Autodesk Inventor part; units mm, degrees
ref_plane "YZ Plane" through (0, 0, 0) normal (1, 0, 0) x (0, 1, 0)
ref_plane "XZ Plane" through (0, 0, 0) normal (0, 1, 0) x (-1, 0, 0)
ref_plane "XY Plane" through (0, 0, 0) normal (0, 0, 1) x (1, 0, 0)
sketch "Sketch1" plane through (0, 0, 0) normal (0, 1, 0) x (-1, 0, 0)
  circle A0 centre (0, 0) radius 7.5
  circle A1 centre (0, -10.775) radius 1.725
  circle A2 centre (0, 10.775) radius 1.725
  line L0 (8.1017, 5.1965) -> (3.205, 12.8307)
  line L1 (-3.205, 12.8307) -> (-8.1017, 5.1965)
  line L2 (-8.1017, -5.1965) -> (-3.205, -12.8307)
  line L3 (3.205, -12.8307) -> (8.1017, -5.1965)
  line L4 (0, -20) -> (0, 18) construction
  arc A3 (-3.205, -12.8307) -> (3.205, -12.8307) centre (0, -10.775) ccw
  arc A4 (8.1017, -5.1965) -> (8.1017, 5.1965) centre (0, 0) ccw
  arc A5 (-8.1017, 5.1965) -> (-8.1017, -5.1965) centre (0, 0) ccw
  arc A6 (3.205, 12.8307) -> (-3.205, 12.8307) centre (0, 10.775) ccw
  dimension "d0" = 15
  dimension "d2" = 3.45
  dimension "d4" = 10.775
  dimension "d8" = 3.45
  dimension "d9" = 10.775
  dimension "d34" = 9.625
  dimension "d35" = 9.625
extrude "Extrusion1" add sketch "Sketch1" along normal blind 1.25 contours A0 | A4 L3 A3 L2 A5 L1 A6 L0
fillet "Fillet1" radius 1.25 8 edges at (5.6534, 1.25, 9.0136) (9.625, 1.25, 0) (5.6534, 1.25, -9.0136) (0, 1.25, -14.5826) (-5.6534, 1.25, -9.0136) (-9.625, 1.25, 0) (-5.6534, 1.25, 9.0136) (0, 1.25, 14.5826)
extrude "Extrusion2" add sketch "Sketch1" against normal blind 11.3 contours A0
fillet "Fillet2" radius 1.25 1 edges at (7.5, -11.3, 0)
sketch "Sketch2" plane through (0, -11.3, 0) normal (0, -1, 0) x (1, 0, 0)
  circle A0 centre (0, 0) radius 3.26 construction
  line L0 (-0.25, -2.26) -> (0.25, -2.26)
  line L1 (0.25, -2.26) -> (0.25, -4.26)
  line L2 (0.25, -4.26) -> (-0.25, -4.26)
  line L3 (-0.25, -4.26) -> (-0.25, -2.26)
  line L4 (-0.25, -2.26) -> (0.25, -4.26) construction
  line L5 (0.25, -2.26) -> (-0.25, -4.26) construction
  circle A1 centre (0, 0) radius 3.26 construction
  line L6 (1.4213, -1.7748) -> (1.7748, -1.4213)
  line L7 (1.7748, -1.4213) -> (3.1891, -2.8355)
  line L8 (3.1891, -2.8355) -> (2.8355, -3.1891)
  line L9 (2.8355, -3.1891) -> (1.4213, -1.7748)
  line L10 (1.4213, -1.7748) -> (3.1891, -2.8355) construction
  line L11 (1.7748, -1.4213) -> (2.8355, -3.1891) construction
  circle A2 centre (0, 0) radius 3.26 construction
  line L12 (2.26, -0.25) -> (2.26, 0.25)
  line L13 (2.26, 0.25) -> (4.26, 0.25)
  line L14 (4.26, 0.25) -> (4.26, -0.25)
  line L15 (4.26, -0.25) -> (2.26, -0.25)
  line L16 (2.26, -0.25) -> (4.26, 0.25) construction
  line L17 (2.26, 0.25) -> (4.26, -0.25) construction
  circle A3 centre (0, 0) radius 3.26 construction
  line L18 (1.7748, 1.4213) -> (1.4213, 1.7748)
  line L19 (1.4213, 1.7748) -> (2.8355, 3.1891)
  line L20 (2.8355, 3.1891) -> (3.1891, 2.8355)
  line L21 (3.1891, 2.8355) -> (1.7748, 1.4213)
  line L22 (1.7748, 1.4213) -> (2.8355, 3.1891) construction
  line L23 (1.4213, 1.7748) -> (3.1891, 2.8355) construction
  circle A4 centre (0, 0) radius 3.26 construction
  line L24 (0.25, 2.26) -> (-0.25, 2.26)
  line L25 (-0.25, 2.26) -> (-0.25, 4.26)
  line L26 (-0.25, 4.26) -> (0.25, 4.26)
  line L27 (0.25, 4.26) -> (0.25, 2.26)
  line L28 (0.25, 2.26) -> (-0.25, 4.26) construction
  line L29 (-0.25, 2.26) -> (0.25, 4.26) construction
  point P0 (0, -3.26)
  point P1 (2.3052, -2.3052)
  point P2 (3.26, 0)
  point P3 (2.3052, 2.3052)
  point P4 (0, 3.26)
  dimension "d16" = 6.52
  dimension "d19" = 0.5
  dimension "d20" = 2
  dimension "d23" = 180
extrude "Extrusion3" add sketch "Sketch2" along normal blind 5
sketch "Sketch3" plane through (0, 1.25, 0) normal (0, 1, 0) x (1, 0, 0)
  arc A0 (-7.0495, 4.5216) -> (-7.0495, -4.5216) centre (0, 0) ccw
  circle A1 centre (0, 0) radius 7.25
  dimension "d27" = 14.5
extrude "Extrusion4" cut sketch "Sketch3" against normal blind 11.25
sketch "Sketch4" plane through (0, -10, 0) normal (0, 1, 0) x (1, 0, 0)
  circle A0 centre (0, 0) radius 5.85
  dimension "d30" = 11.7
extrude "Extrusion5" add sketch "Sketch4" along normal up to surface (11.25 mm away)
fillet "Fillet3" radius 0.5 1 edges at (-7.25, 1.25, 0)
equation "\"d8\" = d2"
equation "\"d35\" = d34"
equation "\"d12\" = d10"
equation "\"d15\" = d10"
properties part number "midi_gniazdo"
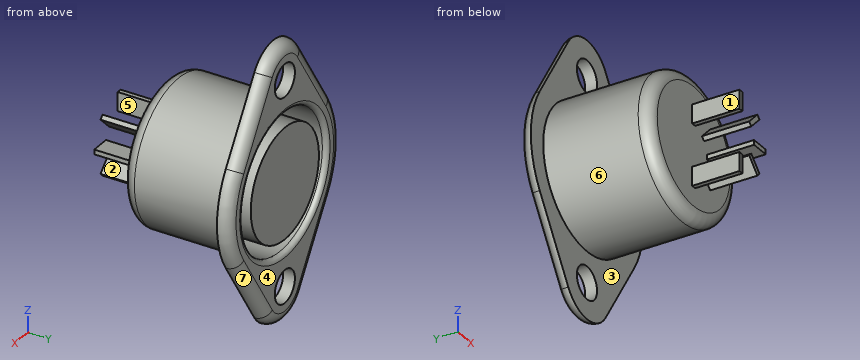
Geometry: final body of the model. Coordinates: model frame, mm. Face numbers are marked on the shaded views. A direction names the side the tool comes from. Give positions to 0.01 mm unless a question says otherwise; leave off trailing zeros. Loops run counter-clockwise (first coordinate to the right, second up) from the corner with the lowest first, then second, coordinate; pieces in that order, holes last. Notation, with made-up numbers: M 55,16 L 76,16 A20 cw 76,26 Z; hole C 84,-5.5 d7. An arc over 180 degrees is marked long. Put each result on its own line as item: value. Start each with the question number.
1) Contact query for flat-ended pins moving along their axis: pin 1 (5 mm diameter, centred on y = -9, z = 7.5, fed in from +X); pin 2 (2 mm diameter, centred on x = 0, z = 10.775, fed in from +Y); pin 3 (0.6 mm diameter, centred on y = -15, z = 0, fed in from -X); pin 4 (5 mm diameter, centred on y = -4.5, z = -3.5, fed in from -X). Output: stop coordinate, or through.
2) Cut plane A-A (y = -3.75). Output: boundary loops of the cut face in (x, z), then the cut area to 3 significant figures.
3) Pull-direction query (X, two-part tool) for the marked faces 4, 5, 6 and 7; classes: pulls with the +X half, pulls with the -X half, needs draft (parallel to the pull), parting line crosses it, or undercut.
4) Ray query, line 1 along X through (y, z) = (-0.75, 0.25); line 2 along Z through (x, y) = (0, -1.5); line 3 along X through (y, z) = (-9.5, -3). Return the intervals inside material, ascending.
5) Cut plane B-B (y = -12.5). Output: boundary loops of the cut face in (x, z).
6) Access query for the marked faces 1, 2 and 3. Directions: +Z, -Z, +X, -X, +Y, -Y. A direction counts if a zero-diameter tool reaches every point of the face in a straight line with its end or side. Return the directions, or none.
Verdict:
1. pin 1: x = 5.59
1. pin 2: through
1. pin 3: x = 2.26
1. pin 4: x = -7.43
2. outline: C 0,0 d15; C 0,0 d11.7; hole C 0,0 d14.5
2. area: 119 mm2
3. face 4: needs draft
3. face 5: undercut
3. face 6: parting line crosses it
3. face 7: pulls with the +X half
4. line 1: -7.5 to -7.25, -5.84 to 5.84, 7.25 to 7.5
4. line 2: -7.5 to -7.25, -5.85 to 5.85, 7.25 to 7.5
4. line 3: -6.87 to -6.6, -5.02 to 5.02, 6.6 to 6.87
5. outline: M -0.25,-4.26 L 0.25,-4.26 L 0.25,-2.26 L -0.25,-2.26 Z; M -0.25,2.26 L 0.25,2.26 L 0.25,4.26 L -0.25,4.26 Z; M 1.42,-1.77 L 2.84,-3.19 L 3.19,-2.84 L 1.77,-1.42 Z; M 1.42,1.77 L 1.77,1.42 L 3.19,2.84 L 2.84,3.19 Z; M 2.26,-0.25 L 4.26,-0.25 L 4.26,0.25 L 2.26,0.25 Z
6. face 1: +Z, -Z, -X, -Y
6. face 2: +X, -Y
6. face 3: -Y
